For this review, take the finished solid that the model builds, in its own axes (mm). Give positions to 0.01 mm unless a question says otherwise; leave off trailing zeros. Loops run counter-clockwise (first coordinate to the right, second up) from the corner with the lowest first, then second, coordinate; pieces in that order, holes last. Notation, with made-up numbers: (-22, 23.25) -> (-5, 23.25) arc R16 ccw to (-5, 43.25) -> close; hole circle Ø5 at (87.5, 89). An arc over 180 degrees is marked (long way). Answer as CSV lines item,"result". Start each with the question number.
Item 1: Add section A-A on z = 873. State the section outline as (x, y) points.
Item 2: Add section B-B on x = 0. State how many separate pieces and enclosed holes the cut face has, plus the area to 3 significant figures.
Item 3: For L1, parallel to X at y = 12.5, z = 630; L2, parallel to X at y = 16.75, z = 607; L3, parallel to X at y = 11.25, z = 711, list the stretches that pass through material, from the lowest coordinate up. Write a range as from..to.
Item 4: Clearance check with flat-ended pins moving along their axes: P1, Ø5, axis at x = 0, z = 770, coming from the +Y side; P2, Ø1, axis at y = 9.5, z = 551.5, coming from the -X side; P3, Ø1, axis at y = 9, z = 382, coming from the +X side. State where each tip first meets the part, or that it passes through.
```python
from build123d import *

# Parameters (mm, degrees)
BOSS_EXTRUDE1_DEPTH = 1400
SKETCH2_R           = 4
CUT_EXTRUDE1_DEPTH  = 26


with BuildPart() as part:
    # Sketch1 → Boss-Extrude1 (new body)
    with BuildSketch(Plane.XY):
        Polygon((-10, 0), (0, 0), (0, 17.5), (-7, 17.5), (-10, 14.5), (-10, 12.5), (-7.75, 10.25), (-7.75, 8.25), (-10, 6), align=None)
        Polygon((0, 17.5), (0, 0), (10, 0), (10, 6), (7.75, 8.25), (7.75, 10.25), (10, 12.5), (10, 14.5), (7, 17.5), align=None)
    extrude(amount=BOSS_EXTRUDE1_DEPTH)

    # Sketch2 → Cut-Extrude1 (cut)
    with BuildSketch(Plane(origin=(0, 17.5, 0), x_dir=(1, 0, 0), z_dir=(0, 1, 0))):
        with Locations(Location((0, -70, 0), (0, 0, 180))):
            Circle(SKETCH2_R)
        with Locations(Location((0, -210, 0), (0, 0, 180))):
            Circle(SKETCH2_R)
        with Locations(Location((0, -350, 0), (0, 0, 180))):
            Circle(SKETCH2_R)
        with Locations(Location((0, -490, 0), (0, 0, 180))):
            Circle(SKETCH2_R)
        with Locations(Location((0, -630, 0), (0, 0, 180))):
            Circle(SKETCH2_R)
        with Locations(Location((0, -770, 0), (0, 0, 180))):
            Circle(SKETCH2_R)
        with Locations(Location((0, -910, 0), (0, 0, 180))):
            Circle(SKETCH2_R)
        with Locations(Location((0, -1050, 0), (0, 0, 180))):
            Circle(SKETCH2_R)
        with Locations(Location((0, -1190, 0), (0, 0, 180))):
            Circle(SKETCH2_R)
        with Locations(Location((0, -1330, 0), (0, 0, 180))):
            Circle(SKETCH2_R)
    extrude(amount=-CUT_EXTRUDE1_DEPTH, mode=Mode.SUBTRACT)


solid = part.part
```
Computed values:
1,outline,"(-10, 0) -> (10, 0) -> (10, 6) -> (7.75, 8.25) -> (7.75, 10.25) -> (10, 12.5) -> (10, 14.5) -> (7, 17.5) -> (-7, 17.5) -> (-10, 14.5) -> (-10, 12.5) -> (-7.75, 10.25) -> (-7.75, 8.25) -> (-10, 6) -> close"
2,separate pieces,"11"
2,enclosed holes,"0"
2,area,"23,100 mm²"
3,L1,"-10..-4, 4..10"
3,L2,"-7.75..7.75"
3,L3,"-8.75..8.75"
4,P1,"through"
4,P2,"x = -7.75"
4,P3,"x = 7.75"
